Autodesk Inventor part; units mm, degrees
ref_plane "Work Plane1" through (28.3459, 0, 0) normal (0, 0, -1) x (-1, 0, 0)
ref_plane "YZ Plane" through (0, 0, 0) normal (1, 0, 0) x (0, 1, 0)
ref_plane "XZ Plane" through (0, 0, 0) normal (0, 1, 0) x (-1, 0, 0)
sketch "Sketch1" plane through (0, 0, 0) normal (0, 0, 1) x (1, 0, 0)
  line L0 (-1.9966, 0) -> (10.6155, 0)
  line L1 (2.9811, 7.1374) -> (1.8959, 9.017)
  line L2 (2.9811, 7.1374) -> (8.8138, 7.1374) construction
  line L3 (8.8138, 7.1374) -> (8.8138, 0) construction
  arc A0 (1.8959, 9.017) -> (0, 8.509) centre (1.016, 8.509) ccw
  line L4 (2.9811, 7.1374) -> (2.9811, 0)
  line L5 (0, -1.9489) -> (0, 11.6933)
  point P0 (0, 0)
  dimension "d2" = 14.2748
  dimension "d4" = 19.05
  dimension "d5" = 1.016
  dimension "d15" = 8.8138
  dimension "d16" = 30
revolve "Ring" add sketch "Sketch1" angle 360 about axis through (-10, 0, 0) along (1, 0, 0)
sketch "Sketch2" plane through (0, 0, 0) normal (-1, 0, 0) x (0, 0, 1)
  circle A0 centre (0, 0) radius 4.9
  line L0 (-7.1374, -4.1208) -> (-7.1374, 4.1208)
  line L1 (-7.1374, 4.1208) -> (0, 8.2416)
  line L2 (0, 8.2416) -> (7.1374, 4.1208)
  line L3 (7.1374, 4.1208) -> (7.1374, -4.1208)
  line L4 (7.1374, -4.1208) -> (0, -8.2416)
  line L5 (0, -8.2416) -> (-7.1374, -4.1208)
  circle A1 centre (0, 0) radius 8.509
  dimension "d6" = 16.4831
extrude "Body" add sketch "Sketch2" against normal blind 8.8138 contours A0 | L0 L1 L2 L3 L4 L5
sketch "Sketch3" plane through (0, 0, 0) normal (0, 0, 1) x (1, 0, 0)
  line L0 (2.3436, 8.2416) -> (8.8138, 8.2416)
  line L1 (8.8138, 4.1208) -> (8.8138, 8.2416)
  line L2 (0, -8.509) -> (0, 8.509)
  line L3 (-1.7628, 0) -> (10.5766, 0)
  line L4 (8.1763, 8.2416) -> (8.8138, 7.1374)
  dimension "d10" = 30
  dimension "d11" = 14.2748
revolve "Chamfer1" cut sketch "Sketch3" angle 360 about axis through (-10, 0, 0) along (1, 0, 0)
sketch "Sketch4" plane through (0, 0, 0) normal (-1, 0, 0) x (0, 0, 1)
  circle A0 centre (0, 0) radius 8.509
hole "Thread" at (0, 0, 0) direction (1, 0, 0) diameter 7.7978 end through all
chamfer "Chamfer2" distance 0.8593 angle 30 1 edges at (0, 0, -3.8989) measured on face at (0, 6.8804, -0.8354)
ref_plane "Work Plane1" through (28.3459, 0, 0) normal (0, 0, -1) x (-1, 0, 0)
chamfer "Chamfer3" distance 0.8593 angle 45 1 edges at (8.8138, 0, -3.8989)
equation "\"d6\" = 1.1547 * SW"
equation "\"d7\" = KOH"
equation "\"d12\" = -0.5 * GD1 + 0.5 * NND"
equation "\"d46\" = -0.5 * GD1 + 0.5 * NND"
equation "\"d51\" = -0.5 * GD1 + 0.5 * NND"
equation "\"d2\" = SW"
equation "\"d4\" = LADI"
equation "\"d5\" = PHH"
equation "\"d15\" = KOH"
equation "\"d16\" = KEWI"
equation "\"d10\" = ANG1"
equation "\"d11\" = SW0"
equation "\"ANG1\" = 30deg"
equation "\"KEWI\" = 30deg"
equation "\"NND\" = 9.525"
equation "\"LADI\" = 19.05"
equation "\"SW\" = 14.2748"
equation "\"PHH\" = 1.016"
equation "\"KOH\" = 8.8138"
equation "\"SW0\" = SW"
equation "\"d1\" = LADI"
equation "\"d3\" = PHH"
equation "\"THREADDIA\" = 9.525"
equation "\"TOA\" = 30deg"
equation "\"E0\" = 1.155 * SW"
properties part number "IFI - I0.375 - 16, HFNI(1)" material "Steel, Mild"
Design review of the part built by this model. Coordinates are the model's own, in mm. A direction names the side the tool comes from. Coordinates: 2 decimals unless noted, no trailing zeros. Write each loop counter-clockwise with the first axis right and the second up, starting at its lowest first coordinate (ties: lowest second). Pieces come first, ordered by that corner, then holes. Notation, with made-up numbers: M 73,12 L 93,12 A14 ccw 93,24 Z; hole C 28.25,-1 d1. An arc over 180 degrees is marked long. Answer as a JSON object with one key per item and string values.
Item 1: Insertion check: pin 1 Ø1.9 at (x, y) = (4.5, 1) entering from +Z; pin 2 Ø1.5 at (x, z) = (6, -1.5) entering from +Y; pin 3 Ø1.9 at (x, y) = (7, -1.5) entering from -Z. Each pin has a flat end and moves straight along its axis. Give the tip position at first contact, or say it passes through.
Outcome:
{"pin 1": "z = 7.14", "pin 2": "y = 7.81", "pin 3": "z = -7.14"}
Item 2: Wall thickness on probe 1 along Z at (x, y) = (6.5, 0); probe 2 along Y at (x, z) = (8.25, 3.5); probe 3 along Z at (x, y) = (2.75, 0): over which ranges is each line inside the solid? List them lowest first.
Outcome:
{"probe 1": "-7.14 to -3.9, 3.9 to 7.14", "probe 2": "-6.22 to -2.31, 2.31 to 6.22", "probe 3": "-7.54 to -3.9, 3.9 to 7.54"}
Item 3: Add section A-A, the plane x = 7.25. Give the boundary of the cut face in (y, z), and give its area (3 significant figures).
Outcome:
{"outline": "M -8.24,0 L -4.12,-7.14 L 4.12,-7.14 L 8.24,0 L 4.12,7.14 L -4.12,7.14 Z; hole C 0,0 d7.8", "area": "129 mm²"}
Item 4: Machinability: for faces 1 (the flat face through (5.53, -6.15, 3.62)), 2 (the flat face through (5.53, -6.21, -3.52)), 3 (the flat face through (5.53, 6.15, -3.62)), 4 (the flat face through (5.53, 6.21, 3.52)), which of the approach directions +Z, -Z, +X, -X, +Y, -Y give a long, thin tool a straight path to every point of the face, cutting with its end or side? Answer none if there is none.
Outcome:
{"face 1": "+Z, +X, -Y", "face 2": "-Z, +X, -Y", "face 3": "-Z, +X, +Y", "face 4": "+Z, +X, +Y"}
